For this review, take the finished solid that the model builds, in its own axes (mm). A direction names the side the tool comes from. Give positions to 0.01 mm unless a question says otherwise; leave off trailing zeros. Order: outer loops, then holes, each group sorted by start corner. A loop starts at its lowest first (then second) coordinate and runs counter-clockwise, first axis right, second up. Notation, with made-up numbers: (41.5, 50) -> (75.5, 50) arc R8 cw to (75.5, 55) -> close; hole circle Ø4 at (1.5, 87.25). An arc over 180 degrees is marked (long way). One line per item, written item: value. Start each with the question number.
Autodesk Inventor part; units mm, degrees
ref_plane "Work Plane1" through (0, 0, 0) normal (-1, 0, 0) x (0, 0, 1)
ref_plane "YZ Plane" through (0, 0, 0) normal (1, 0, 0) x (0, 1, 0)
ref_plane "XZ Plane" through (0, 0, 0) normal (0, 1, 0) x (-1, 0, 0)
sketch "Sketch1" plane through (0, 0, 0) normal (1, 0, 0) x (0, 1, 0)
  line L0 (-15, 15) -> (15, 15)
  line L1 (15, 15) -> (15, -15)
  line L2 (15, -15) -> (-15, -15)
  line L3 (-15, -15) -> (-15, 15)
  line L4 (-15, 15) -> (15, -15) construction
  line L5 (15, 15) -> (-15, -15) construction
  point P0 (0, 0)
  dimension "d0" = 30
  dimension "d1" = 30
extrude "Extrusion1" add sketch "Sketch1" along normal blind 1.7695
sketch "Sketch2" plane through (1.7695, 0, 0) normal (1, 0, 0) x (0, 0, -1)
  circle A0 centre (0, 0) radius 12
  dimension "d4" = 24
extrude "Extrusion2" cut sketch "Sketch2" against normal up to next
sketch "Sketch3" plane through (0, 0, 0) normal (0, 0, 1) x (1, 0, 0)
  line L0 (1.7695, 15) -> (1.7695, -15)
  line L1 (1.7695, 0) -> (1.7695, -12.5584)
  line L2 (0.5, 0) -> (1.7695, 0)
  arc A0 (0.5, 0) -> (1.7695, -12.5584) centre (63.25, 0) ccw
  point P0 (0, 0)
  dimension "d7" = 12.5584
  dimension "d8" = 125.5
revolve "Revolution1" cut sketch "Sketch3" angle 360 about axis through (0.5, 0, 0) along (1, 0, 0)
sketch "Sketch4" plane through (1.7695, 0, 0) normal (1, 0, 0) x (0, 0, -1)
  circle A0 centre (0, 0) radius 12.7
  line L0 (-15, 15) -> (-15, -15)
  line L1 (-15, 15) -> (15, 15)
  line L2 (15, 15) -> (15, -15)
  line L3 (15, -15) -> (-15, -15)
  line L4 (-15, -15) -> (-15, 15)
  dimension "d10" = 25.4
extrude "Extrusion3" add sketch "Sketch4" along normal blind 3
ref_plane "Work Plane1" through (0, 0, 0) normal (-1, 0, 0) x (0, 0, 1)
mirror "Mirror1" about plane through (0, 0, 0) normal (-1, 0, 0) of "Extrusion1", "Extrusion2", "Revolution1", "Extrusion3"
sketch "Sketch8" plane through (4.7695, 0, 0) normal (1, 0, 0) x (0, 0, -1)
  circle A0 centre (12, -12) radius 1.5
  line L0 (-15, -15) -> (15, -15)
  line L1 (15, -15) -> (15, 15)
  circle A1 centre (-12, -12) radius 1.5
  circle A2 centre (-12, 9) radius 1.5
  line L2 (-15, 15) -> (-15, -15)
  line L3 (15, 15) -> (-15, 15)
  point P0 (0, 0)
  dimension "d30" = 3
  dimension "d31" = 3
  dimension "d32" = 3
  dimension "d33" = 3
  dimension "d34" = 3
  dimension "d35" = 3
  dimension "d36" = 6
extrude "Extrusion7" cut sketch "Sketch8" against normal up to surface (9.5391 mm away) contours A0 | A1 | A2
sketch "Sketch9" plane through (4.7695, 0, 0) normal (1, 0, 0) x (0, 0, -1)
  line L0 (0, 0) -> (-8.2274, 11.75)
  line L1 (-8.2274, 11.75) -> (-15, 11.75)
  line L2 (-15, 15) -> (-15, -15)
  line L3 (0, 0) -> (0, 15) construction
  line L4 (-15, 11.75) -> (-15, 15)
  line L5 (15, 15) -> (-15, 15)
  line L6 (0, 15) -> (-15, 15)
  line L7 (0, 0) -> (8.2274, 11.75)
  line L8 (8.2274, 11.75) -> (15, 11.75)
  line L9 (15, 15) -> (15, -15)
  line L10 (-15, 15) -> (15, 15)
  dimension "d39" = 35
  dimension "d42" = 3.25
extrude "Extrusion8" cut sketch "Sketch9" against normal up to surface (9.5391 mm away)
sketch "Sketch11" plane through (4.7695, -15, -15) normal (0, 0, -1) x (-1, 0, 0)
  line L0 (9.5391, 0) -> (9.5391, 26.75)
  line L1 (0, 0) -> (9.5391, 26.75) construction
  line L2 (0, 26.75) -> (9.5391, 26.75)
  line L3 (0, 26.75) -> (9.5391, 0) construction
  line L4 (0, 0) -> (0, 26.75)
  line L5 (9.5391, 3.375) -> (0, 3.375)
  line L6 (0, 3.375) -> (0, 23.375)
  line L7 (0, 23.375) -> (9.5391, 23.375)
  line L8 (9.5391, 23.375) -> (9.5391, 3.375)
  line L9 (9.5391, 3.375) -> (0, 23.375) construction
  line L10 (0, 3.375) -> (9.5391, 23.375) construction
  point P0 (4.7695, 15)
  point P1 (4.7695, 13.375)
  dimension "d46" = 20
extrude "Extrusion10" add sketch "Sketch11" along normal blind 10 contours L5 L4 L7 L0
sketch "Sketch12" plane through (-4.7695, -15, -15) normal (-1, 0, 0) x (0, 0, 1)
  circle A0 centre (-5, 19.375) radius 1.5
  circle A1 centre (-5, 7.375) radius 1.5
  line L0 (0, 3.375) -> (-10, 3.375)
  line L1 (0, 23.375) -> (-10, 23.375)
  point P0 (15, 15)
  dimension "d49" = 4
  dimension "d50" = 5
  dimension "d51" = 4
  dimension "d52" = 5
  dimension "d53" = 3
extrude "Extrusion11" cut sketch "Sketch12" against normal up to surface (9.5391 mm away)
sketch "Sketch13" plane through (4.7695, -15, -15) normal (0, -1, 0) x (1, 0, 0)
  line L0 (-9.5391, 30) -> (0, 30)
  line L1 (-4.7695, 30) -> (-4.7695, -10)
  line L2 (0, -10) -> (-9.5391, -10)
  point P0 (-4.7695, 15)
split body "Split2" sketch "Sketch13" result one side removed curves L1 removed pieces at (-0.5, -13.971, -0.4809)
equation "\"d37\" = d32"
properties part number "LargeLensHolderP1S1" material "Acetal Resin, Black"
Q1. Mouldability with a two-part tool opening along Z and no side actions: class faces 1 (the flat face through (2.4, 11, 7.7)), 2 (the flat face through (2, -2, 15)), 3 (the flat face through (2, 8.375, -20)) as pulls with the +Z half, pulls with the -Z half, needs draft (parallel to the pull), parting line crosses it, or undercut.
Q2. For line 1 along Y through (x, z) = (2.05, -20) (3 decimals); line 2 along Z through (x, y) = (4.35, -11.75); line 3 along Z through (x, y) = (1.1, 0), list the stretches that pass through material, from the lowest coordinate up.
Q3. Take a section at B-B (x = 3.7). State the section outline as (y, z) points (3 decimals).
Q4. For pin 1 Ø3.5 at (y, z) = (-12, -12) entering from -X; pin 2 Ø1 at (y, z) = (-8.5, 8) entering from +X, all flat-tipped, find the tip position at first contact; note any pin that passes through.
Q5. Take a section at C-C (y = -7). State how many separate pieces and enclosed holes the cut face has, and give its area (3 significant figures).
Q6. Take a section at A-A (z = -20). State the section outline as (x, y) points (1 decimal).
Q7. For faces 4 (the cylindrical face through (3.248, -12.692, -0.45)), 5 (the flat face through (2, 10, -15)), 6 (the flat face through (2, -11.625, -20)), list the 3-axis set-ups (+Z, -Z, +X, -X, +Y, -Y) from which the entire face can be reached by the end or side of a thin tool; tool diameter is ignored.
Answers below:
1. face 1: undercut
1. face 2: pulls with the +Z half
1. face 3: needs draft
2. line 1: y = -11.625 to -9.125, -6.125 to 2.875, 5.875 to 8.375
2. line 2: z = -15 to -13.48, -10.52 to -4.82, 4.82 to 10.52, 13.48 to 15
2. line 3: z = -25 to -12, 12 to 15
3. outline: (-15, -15) -> (-11.625, -15) -> (-11.625, -25) -> (8.375, -25) -> (8.375, -15) -> (11.75, -15) -> (11.75, -8.227) -> (10.403, -7.284) arc R12.7 cw (long way) to (10.403, 7.284) -> (11.75, 8.227) -> (11.75, 15) -> (-15, 15) -> close; hole circle Ø3 at (-12, -12); hole circle Ø3 at (-12, 12); hole circle Ø3 at (-7.625, -20); hole circle Ø3 at (4.375, -20); hole circle Ø3 at (9, 12)
4. pin 1: stops at x = 0
4. pin 2: stops at x = 1.69
5. separate pieces: 3
5. enclosed holes: 0
5. area: 79.6 mm²
6. outline: (0, -11.6) -> (4.8, -11.6) -> (4.8, -9.1) -> (0, -9.1) -> close; (0, -6.1) -> (4.8, -6.1) -> (4.8, 2.9) -> (0, 2.9) -> close; (0, 5.9) -> (4.8, 5.9) -> (4.8, 8.4) -> (0, 8.4) -> close
7. face 4: +X
7. face 5: -Z, +X, -X, +Y
7. face 6: -Z, +X, -X, -Y
